```python
from build123d import *

# Parameters (mm, degrees)
SKETCH2_W                 = 35.56
SKETCH2_H                 = 5.08
BOSS_EXTRUDE1_DEPTH       = 7.62
SKETCH7_W                 = 8.89
SKETCH7_H                 = 6.096
SKETCH7_H_2               = 1.016
CUT_EXTRUDE2_DEPTH        = 6.08
CUT_EXTRUDE3_REACH        = 9.62
SKETCH8_R                 = 2.159
SKETCH9_R                 = 2.159
CUT_EXTRUDE4_DEPTH        = 7.604
F_6_32_TAPPED_HOLE1_D     = 2.7051
F_6_32_TAPPED_HOLE1_DEPTH = 0.762


with BuildPart() as part:
    # Sketch2 → Boss-Extrude1 (new body)
    with BuildSketch(Plane.XY):
        with Locations((-54.739863719, -4.815217495)):
            Rectangle(SKETCH2_W, SKETCH2_H)
    extrude(amount=BOSS_EXTRUDE1_DEPTH)

    # Sketch7 → Cut-Extrude2 (cut, through all)
    with BuildSketch(Plane.XZ.offset(7.355217495)):
        with Locations((-41.404863719, 3.81)):
            Rectangle(SKETCH7_W, SKETCH7_H)
        with Locations((-68.074863719, 0.508)):
            Rectangle(SKETCH7_W, SKETCH7_H_2)
        with Locations((-68.074863719, 7.112)):
            Rectangle(SKETCH7_W, SKETCH7_H_2)
    extrude(amount=-CUT_EXTRUDE2_DEPTH, mode=Mode.SUBTRACT)

    # Sketch8 → Cut-Extrude3 (cut, up to next)
    with BuildSketch(Plane.XY.offset(7.62), mode=Mode.PRIVATE) as cut_extrude3_sk1:
        with Locations((-40.769863719, -4.815217495)):
            Circle(SKETCH8_R)
    cut_extrude3_tool1 = extrude(cut_extrude3_sk1.sketch, amount=-CUT_EXTRUDE3_REACH, mode=Mode.PRIVATE) & part.part
    add(cut_extrude3_tool1.solids().sort_by_distance((-40.769864, -4.815217, 7.62))[0], mode=Mode.SUBTRACT)

    # Sketch9 → Cut-Extrude4 (cut, through all)
    with BuildSketch(Plane.XY.offset(6.604)):
        with Locations((-68.963863719, -4.815217495)):
            Circle(SKETCH9_R)
    extrude(amount=-CUT_EXTRUDE4_DEPTH, mode=Mode.SUBTRACT)

    # #6-32 Tapped Hole1
    with Locations(Plane(origin=(0, 0, 0), x_dir=(-1, 0, 0), z_dir=(0, 0, -1))):
        with Locations((40.769863719, -4.815217495)):
            Hole(F_6_32_TAPPED_HOLE1_D / 2, depth=F_6_32_TAPPED_HOLE1_DEPTH)


solid = part.part
```
The listing builds one solid part. Answer for the finished solid, in the listing's coordinates (mm). A direction names the side the tool comes from. Coordinates: 2 decimals unless noted, no trailing zeros. Loops run counter-clockwise (first coordinate to the right, second up) from the corner with the lowest first, then second, coordinate; pieces in that order, holes last. Notation, with made-up numbers: M 68,37 L 107,37 A24 ccw 107,61 Z; hole C -23.75,22 d5. An arc over 180 degrees is marked long. Answer as a JSON object with one key per item and string values. Group by question number.
Item 1: Section B-B (y = -6.55) is taken. Write down the section's boundary in (x, z), and give its area (3 significant figures).
Item 2: Section D-D (y = -4.1) is taken. Write down the section's boundary in (x, z), and give its area (3 significant figures).
Item 3: Section A-A (x = -44) is taken. Write down the section's boundary in (y, z), and give its area (3 significant figures).
Item 4: Each of these flat-tipped pins is pushed along its axis until it touches: P1, Ø1.5, axis at y = -5, z = 2.5, coming from the +X side; P2, Ø0.5, axis at y = -5.5, z = 7, coming from the -X side; P3, Ø2, axis at x = -40.77, y = -4.82, coming from the -Z side. Where does it stop, or does it pass through?
Item 5: Which of the six approach directions +Z, -Z, +X, -X, +Y, -Y give full straight-line access (tool end or side, diameter ignored) to faces 4 (the face through (-42.5, -4.9, 0.762)), 5 (the face through (-66, -5, 1.016)), 6 (the face through (-42.927, -4.72, 7.244)), 7 (the face through (-66, -5, 6.604))?
Item 6: Consider L1, parallel to Z at x = -41, y = -2.5; L2, parallel to X at y = -4.8, z = 1.5; L3, parallel to X at y = -6.45, z = 0.5. Determine where each line is inside the solid, lowest interval first.
Item 7: Section C-C (z = 6.25) is taken. Write down the section's boundary in (x, y), and give its area (3 significant figures).
Item 8: Determine the mould class of faces 1 (the face through (-59, -7.355, 4)), 2 (the face through (-45.85, -5, 4)), 3 (the face through (-50, -5, 0)) for opening direction Z: +Z half, -Z half, draft (parallel to the pull), parting line (faces both ways), or undercut.
Solved:
{
 "1": {"outline": "M -72.52,1.02 L -70.25,1.02 L -70.25,6.6 L -72.52,6.6 Z; M -67.68,1.02 L -63.63,1.02 L -63.63,0 L -36.96,0 L -36.96,0.76 L -45.85,0.76 L -45.85,6.86 L -42.06,6.86 L -42.06,7.62 L -63.63,7.62 L -63.63,6.6 L -67.68,6.6 Z; M -39.48,6.86 L -36.96,6.86 L -36.96,7.62 L -39.48,7.62 Z", "area": "182 mm2"},
 "2": {"outline": "M -72.52,1.02 L -71,1.02 L -71,6.6 L -72.52,6.6 Z; M -66.93,1.02 L -63.63,1.02 L -63.63,0 L -41.92,0 L -41.92,0.76 L -45.85,0.76 L -45.85,6.86 L -42.81,6.86 L -42.81,7.62 L -63.63,7.62 L -63.63,6.6 L -66.93,6.6 Z; M -39.62,0 L -36.96,0 L -36.96,0.76 L -39.62,0.76 Z; M -38.73,6.86 L -36.96,6.86 L -36.96,7.62 L -38.73,7.62 Z", "area": "171 mm2"},
 "3": {"outline": "M -7.36,0 L -2.28,0 L -2.28,0.76 L -7.36,0.76 Z; M -7.36,6.86 L -2.28,6.86 L -2.28,7.62 L -7.36,7.62 Z", "area": "7.74 mm2"},
 "4": {"P1": "stops at x = -45.85", "P2": "stops at x = -63.63", "P3": "passes through"},
 "5": {"face 4": "+X, +Y, -Y", "face 5": "-Z, -X, +Y, -Y", "face 6": "+Z", "face 7": "+Z, -X, +Y, -Y"},
 "6": {"L1": "z = 0 to 0.76, 6.86 to 7.62", "L2": "x = -72.52 to -71.12, -66.8 to -45.85", "L3": "x = -63.63 to -36.96"},
 "7": {"outline": "M -72.52,-7.36 L -45.85,-7.36 L -45.85,-2.28 L -72.52,-2.28 Z; hole C -68.96,-4.82 d4.32", "area": "121 mm2"},
 "8": {"face 1": "draft", "face 2": "undercut", "face 3": "-Z half"}
}
